For this review, take the finished solid that the model builds, in its own axes (mm). Give positions to 0.01 mm unless a question says otherwise; leave off trailing zeros.
```python
from build123d import *

# Parameters (mm, degrees)
SKETCH1_W               = 76.2
SKETCH1_H               = 152.4
BOSS_EXTRUDE1_DEPTH     = 6.35
F_1_4_CLEARANCE_HOLE1_D = 6.7564


with BuildPart() as part:
    # Sketch1 → Boss-Extrude1 (new body)
    with BuildSketch(Plane.XY):
        Rectangle(SKETCH1_W, SKETCH1_H)
    extrude(amount=BOSS_EXTRUDE1_DEPTH)

    # 1/4 Clearance Hole1 (through all)
    with Locations(Plane.XY.offset(6.35)):
        with Locations((-28.575, 66.675), (28.575, 66.675)):
            f_1_4_clearance_hole1 = Hole(F_1_4_CLEARANCE_HOLE1_D / 2)

    # Mirror1: 1/4 Clearance Hole1 across plane
    add(f_1_4_clearance_hole1.mirror(Plane.ZX), mode=Mode.SUBTRACT)


solid = part.part
```
Q1. For probe 1 along X at (y, z) = (-67, 1.5); probe 2 along Y at (x, z) = (-30, 3.75); probe 3 along Y at (x, z) = (-25.5, 1), list the stretches that pass through material, from the lowest coordinate up.
Answers:
probe 1: x = -38.1 to -31.94, -25.21 to 25.21, 31.94 to 38.1
probe 2: y = -76.2 to -69.74, -63.61 to 63.61, 69.74 to 76.2
probe 3: y = -76.2 to -68.07, -65.28 to 65.28, 68.07 to 76.2
Q2. For pin 1 Ø5.5 at (x, y) = (-28.575, -66.675) entering from -Z, flat-tipped, find the tip position at first contact; note if it passes through.
Answers:
pin 1: passes through
Q3. Mouldability with a two-part tool opening along X and no side actions: class faces 1 (the cylindrical face through (-30.391, -69.524, 3.131)), 2 (the flat face through (-38.1, -1, 3)), 3 (the flat face through (-1, 1, 6.35)) as +X half, -X half, draft (parallel to the pull), parting line (faces both ways), or undercut.
Answers:
face 1: undercut
face 2: -X half
face 3: draft
